from build123d import *

# Parameters (mm, degrees)
F0_R     = 70
F1_DEPTH = 20
F2_R     = 15
F3_W     = 25
F3_H     = 120


with BuildPart() as f1:
    # F0 (on Front) → F1 (new body, symmetric)
    with BuildSketch(Plane.XZ):
        Circle(F0_R)
    extrude(amount=F1_DEPTH, both=True)

    # F2
    f2_edges = [f1.edges().sort_by_distance(p)[0] for p in [
        (-70, -20, 0),
        (-70, 20, 0),
    ]]
    fillet(f2_edges, radius=F2_R)

    # F3 (on Front) → F4 (revolve)
    with BuildSketch(Plane.XZ):
        with Locations((-12.5, 60)):
            Rectangle(F3_W, F3_H)
    revolve(axis=Axis((0, 0, 60), (0, 0, 1)))


solid = f1.part
Part model, mm, in its own coordinate system. A direction names the side the tool comes from. Coordinates: 2 decimals unless noted, no trailing zeros. Order: outer loops, then holes, each group sorted by start corner. A loop starts at its lowest first (then second) coordinate and runs counter-clockwise, first axis right, second up. Notation, with made-up numbers: M 54.25,25.25 L 68.25,25.25 A13 cw 68.25,50.25 Z; hole C 48.25,45.5 d7. An arc over 180 degrees is marked long. Use a Markdown table: item, result.
(1) Tool access for faces 1 (the flat face through (0, -22, 0)), 2 (the flat face through (0, 22, 0)), 3 (the flat face through (-1, -20, -12)): list every direction of +Z, -Z, +X, -X, +Y, -Y with a clear straight run to the whole face (end or side of a thin tool).
A:
| item | result |
|---|---|
| face 1 | -Z, +X, -X, -Y |
| face 2 | -Z, +X, -X, +Y |
| face 3 | -Z, -Y |
(2) Probe L1, parallel to Y at x = -4, z = -17.5; L2, parallel to X at y = -4, z = 1.5; L3, parallel to Y at x = -1.5, z = 43.5. List the from-to ranges inside material, lowest first.
A:
| item | result |
|---|---|
| L1 | y = -20 to 20 |
| L2 | x = -69.98 to 69.98 |
| L3 | y = -24.95 to 24.95 |
(3) Cut at D-D on y = 0. Write the cut outline in (x, z), then the cut area to 3 significant figures.
A:
| item | result |
|---|---|
| outline | M -25,65.38 A70 ccw long 25,65.38 L 25,120 L -25,120 Z |
| area | 18,000 mm^2 |
(4) Cut at C-C on y = -13.5. Write the cut outline in (x, z).
A:
| item | result |
|---|---|
| outline | M -21.04,63.99 A67.36 ccw long 21.04,63.99 L 21.04,120 L -21.04,120 Z |
(5) Flat gauge pins, fed straight in: pin 1 (1.5 mm diameter, centred on x = 3.5, y = -23, fed in from -Z); pin 2 (1.5 mm diameter, centred on x = -36.5, z = 33, fed in from +Y); pin 3 (5 mm diameter, centred on x = 21.5, z = 63, fed in from -Y); pin 4 (1 mm diameter, centred on x = 56, z = 43.5, fed in from +Y). Where does each tip first touch, or does it go through?
A:
| item | result |
|---|---|
| pin 1 | stops at z = 0 |
| pin 2 | stops at y = 20 |
| pin 3 | stops at y = -16.95 |
| pin 4 | passes through |
(6) Cut at B-B on z = 70.5. Write the cut outline in (x, y).
A:
| item | result |
|---|---|
| outline | C 0,0 d50 |
(7) Cut at A-A on x = 0. Write the cut outline in (y, z).
A:
| item | result |
|---|---|
| outline | M -25,0 L -20,0 L -20,-55 A15 ccw -5,-70 L 5,-70 A15 ccw 20,-55 L 20,0 L 25,0 L 25,120 L -25,120 Z |
